Check sheet for the modelled part. Datum: model origin and axes. Units: mm. Give positions to 0.01 mm unless a question says otherwise; leave off trailing zeros. Order: outer loops, then holes, each group sorted by start corner. A loop starts at its lowest first (then second) coordinate and runs counter-clockwise, first axis right, second up. Notation, with made-up numbers: (40.5, -39.5) - (57.5, -39.5) arc R29 cw to (57.5, -14.5) - close; hole circle Ø9 at (72, -22.5). An arc over 180 degrees is marked (long way). Answer in a Markdown table with one row per item.
from build123d import *

# Parameters (mm, degrees)
F0_W     = 31.5
F0_H     = 48
F0_R     = 1.95
F0_R_2   = 14
F1_DEPTH = 1.2


with BuildPart() as f1:
    # F0 (on Front) → F1 (new body)
    with BuildSketch(Plane.XZ):
        with Locations((0, -1)):
            Rectangle(F0_W, F0_H)
        with Locations((-10.75, -20)):
            Circle(F0_R, mode=Mode.SUBTRACT)
        with Locations((10.75, -20)):
            Circle(F0_R, mode=Mode.SUBTRACT)
        with Locations((0, -4)):
            Circle(F0_R_2, mode=Mode.SUBTRACT)
        with Locations((-10.75, 18)):
            Circle(F0_R, mode=Mode.SUBTRACT)
        with Locations((10.75, 18)):
            Circle(F0_R, mode=Mode.SUBTRACT)
    extrude(amount=F1_DEPTH)


solid = f1.part
(1) Cross-section at B-B, the plane y = -0.3. Record the cut outline in (x, z), then the cut area to 3 significant figures.
Geometry says:
| item | result |
|---|---|
| outline | (-15.75, -25) - (15.75, -25) - (15.75, 23) - (-15.75, 23) - close; hole circle Ø28 at (0, -4); hole circle Ø3.9 at (-10.75, -20); hole circle Ø3.9 at (-10.75, 18); hole circle Ø3.9 at (10.75, -20); hole circle Ø3.9 at (10.75, 18) |
| area | 848 mm² |
(2) Mould release check, pull along X, two halves, no side actions. Record for faces 1 (the cylindrical face through (-9.85, -0.59, -21.73)), 2 (the flat face through (-15.75, -1, -1)), 3 (the flat face through (-4, -1.2, 10)): pulls with the +X half, pulls with the -X half, needs draft (parallel to the pull), parting line crosses it, or undercut.
Geometry says:
| item | result |
|---|---|
| face 1 | undercut |
| face 2 | pulls with the -X half |
| face 3 | needs draft |
(3) Cross-section at C-C, the plane z = -20. Record the cut outline in (x, y).
Geometry says:
| item | result |
|---|---|
| outline | (-15.75, -1.2) - (-12.7, -1.2) - (-12.7, 0) - (-15.75, 0) - close; (-8.8, -1.2) - (8.8, -1.2) - (8.8, 0) - (-8.8, 0) - close; (12.7, -1.2) - (15.75, -1.2) - (15.75, 0) - (12.7, 0) - close |
(4) Thickness scan on L1, parallel to Z at x = -0.5, y = -0.4; L2, parallel to Z at x = -9.5, y = -0.8; L3, parallel to Z at x = -9, y = -0.35. Record the ranges inside material, lowest first.
Geometry says:
| item | result |
|---|---|
| L1 | -25 to -17.99, 9.99 to 23 |
| L2 | -25 to -21.5, -18.5 to -14.28, 6.28 to 16.5, 19.5 to 23 |
| L3 | -25 to -20.86, -19.14 to -14.72, 6.72 to 17.14, 18.86 to 23 |
(5) Cross-section at D-D, the plane z = 5.5. Record the cut outline in (x, y), then the cut area to 3 significant figures.
Geometry says:
| item | result |
|---|---|
| outline | (-15.75, -1.2) - (-10.28, -1.2) - (-10.28, 0) - (-15.75, 0) - close; (10.28, -1.2) - (15.75, -1.2) - (15.75, 0) - (10.28, 0) - close |
| area | 13.1 mm² |
(6) Cross-section at A-A, the plane x = 0. Record the cut outline in (y, z).
Geometry says:
| item | result |
|---|---|
| outline | (-1.2, -25) - (0, -25) - (0, -18) - (-1.2, -18) - close; (-1.2, 10) - (0, 10) - (0, 23) - (-1.2, 23) - close |
